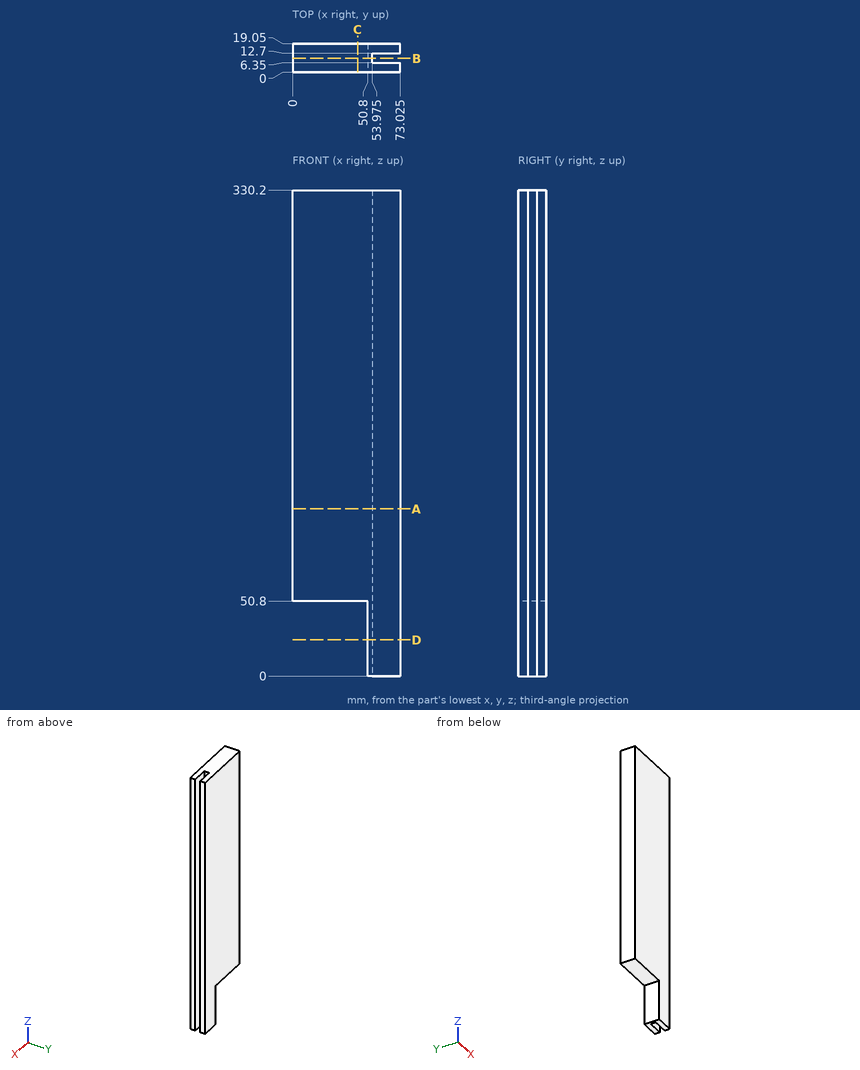
The drawing under review shows one solid part. Ordinate dimensions are in mm from its lowest x, y, z. Coordinates: 2 decimals unless noted, no trailing zeros. Write each loop counter-clockwise with the first axis right and the second up, starting at its lowest first coordinate (ties: lowest second). Pieces come first, ordered by that corner, then holes. Notation, with made-up numbers: (11, 16) - (24, 16) arc R9 cw to (24, 21) - close; hole circle Ø1 at (31.5, 51.25). An arc over 180 degrees is marked (long way). Answer in a Markdown table with one row per item. Add a question column.
Q1. We need section A-A, the plane z = 113.5. State the section outline as (x, y) points (3 decimals).
Q2. For P1, Ø12, axis at x = 63, z = 275.5, coming from the -Y side; P2, Ø5.5, axis at y = 10, z = 36.5, coming from the -X side; P3, Ø5.5, axis at x = 14.5, y = 12.5, coming from the -Z side, all flat-tipped, find the tip position at first contact; note any pin that passes through.
Q3. We need section D-D, the plane z = 24.5. State the section outline as (x, y) points (3 decimals), and give its area (3 significant figures).
Q4. For probe 1 along Y at (x, z) = (64, 315.5); probe 2 along Z at (x, y) = (14, 8.25); probe 3 along X at (y, z) = (5.75, 38) (3 decimals), list the stretches that pass through material, from the lowest coordinate up.
Q5. We need section C-C, the plane x = 44. State the section outline as (y, z) points.
Q6. We need section B-B, the plane y = 9.25. State the section outline as (x, z) points (3 decimals).
Answer list:
| question | item | result |
|---|---|---|
| 1 | outline | (0, 0) - (73.025, 0) - (73.025, 6.35) - (53.975, 6.35) - (53.975, 12.7) - (73.025, 12.7) - (73.025, 19.05) - (0, 19.05) - close |
| 2 | P1 | stops at y = 0 |
| 2 | P2 | stops at x = 50.8 |
| 2 | P3 | stops at z = 50.8 |
| 3 | outline | (50.8, 0) - (73.025, 0) - (73.025, 6.35) - (53.975, 6.35) - (53.975, 12.7) - (73.025, 12.7) - (73.025, 19.05) - (50.8, 19.05) - close |
| 3 | area | 302 mm2 |
| 4 | probe 1 | y = 0 to 6.35, 12.7 to 19.05 |
| 4 | probe 2 | z = 50.8 to 330.2 |
| 4 | probe 3 | x = 50.8 to 73.025 |
| 5 | outline | (0, 50.8) - (19.05, 50.8) - (19.05, 330.2) - (0, 330.2) - close |
| 6 | outline | (0, 50.8) - (50.8, 50.8) - (50.8, 0) - (53.975, 0) - (53.975, 330.2) - (0, 330.2) - close |
